Autodesk Inventor part; units mm, degrees
ref_plane "YZ Plane" through (0, 0, 0) normal (1, 0, 0) x (0, 1, 0)
ref_plane "XZ Plane" through (0, 0, 0) normal (0, 1, 0) x (-1, 0, 0)
ref_plane "XY Plane" through (0, 0, 0) normal (0, 0, 1) x (1, 0, 0)
sketch "Sketch1" plane through (0, 0, 0) normal (0, 0, 1) x (1, 0, 0)
  line L0 (0, 0) -> (25.4, 0)
  line L1 (25.4, 0) -> (25.4, 25.4)
  line L2 (25.4, 25.4) -> (0, 25.4)
  line L3 (0, 25.4) -> (0, 0)
  line L4 (1.5875, 1.5875) -> (23.8125, 1.5875)
  line L5 (23.8125, 1.5875) -> (23.8125, 23.8125)
  line L6 (23.8125, 23.8125) -> (1.5875, 23.8125)
  line L7 (1.5875, 23.8125) -> (1.5875, 1.5875)
  dimension "d0" = 25.4
  dimension "d1" = 25.4
  dimension "d2" = 1.5875
extrude "Extrusion1" add sketch "Sketch1" along normal blind 400.05
sketch "Sketch3" plane through (0, 25.4, 0) normal (0, 1, 0) x (1, 0, 0)
  line L0 (25.4, 0) -> (0, 0)
  line L1 (0, 0) -> (0, -400.05)
  line L2 (25.4, -400.05) -> (0, -400.05)
  line L3 (25.4, 0) -> (25.4, -400.05)
  point P0 (0, 0)
  point P1 (12.7, -200.025)
  dimension "d15" = 200.025
  dimension "d16" = 400.05
  dimension "d17" = 12.7
hole "Hole2" at (12.7, 25.4, 200.025) direction (0, -1, 0) diameter 6.35 end through all
sketch "Sketch7" plane through (0, 25.4, 0) normal (0, 1, 0) x (1, 0, 0)
  line L0 (0, 0) -> (0, -400.05)
  line L1 (25.4, 0) -> (25.4, -400.05)
  line L2 (25.4, 0) -> (0, 0)
  line L3 (0, 0) -> (25.4, 0)
  line L4 (0, -200.025) -> (0, 0)
  line L5 (25.4, 0) -> (25.4, -200.025)
  line L6 (0, 0) -> (25.4, 0)
  arc A0 (25.4, -200.025) -> (0, -200.025) centre (12.7, -200.025) ccw
  line L7 (25.4, -400.05) -> (0, -400.05)
  circle A1 centre (12.7, -200.025) radius 3.175
  line L8 (25.4, 0) -> (0, 0)
  line L9 (0, 0) -> (0, -400.05)
  line L10 (25.4, -400.05) -> (0, -400.05)
  line L11 (25.4, 0) -> (25.4, -400.05)
extrude "Extrusion3" cut sketch "Sketch7" against normal blind 25.4 contours L2 L1 A0 L0
sketch "Sketch8" plane through (0, 25.4, 400.05) normal (0, 1, 0) x (1, 0, 0)
  line L0 (25.4, 0) -> (0, 0)
  line L1 (0, 200.025) -> (0, 0)
  point P0 (0, 400.05)
  point P1 (12.7, 12.7)
  point P2 (12.7, 31.75)
  point P3 (12.7, 50.8)
  dimension "d43" = 12.7
  dimension "d44" = 12.7
  dimension "d55" = 19.05
  dimension "d56" = 19.05
hole "Hole4" at (12.7, 25.4, 387.35) at (12.7, 25.4, 368.3) at (12.7, 25.4, 349.25) direction (0, -1, 0) diameter 4.8514 end through all
properties part number "CLB_036_FourPartScissorBarTop" material "Aluminum 6061"
Read the model definition and answer for the solid it produces. Units are mm, in the model's axes. A direction names the side the tool comes from. Round coordinates to 2 decimals unless told otherwise and drop trailing zeros. Order: outer loops, then holes, each group sorted by start corner. A loop starts at its lowest first (then second) coordinate and runs counter-clockwise, first axis right, second up.
1) For faces 1 (the face through (13, 1.588, 292)), 2 (the face through (13, 25.4, 292)), determine the directions among +Z, -Z, +X, -X, +Y, -Y from which every point of the face is accessible in a straight line to the end or side of a thin tool.
2) The mould has two halves that part along Z. Classify faces 3 (the face through (1, 13, 400.05)), 4 (the face through (12.593, 0.783, 384.927)), 5 (the face through (1.588, 13, 296)), 6 (the face through (25.253, 15.7, 198.095)): released by +Z, released by -Z, zero draft, split by the parting line, or undercut.
3) A flat-ended cylindrical pin translates along its axis: pin 1 (3 mm diameter, centred on x = 17, y = 5, fed in from +Z). Find the tip coordinate at first contact, or state that the pin passes through.
4) The part is cut by section B-B on z = 344. Write down the section's boundary in (x, y).
5) The part is cut by section C-C on x = 12.7. Give the number of separate pieces and of enclosed holes in the cut face, plus the area to 3 significant figures.
6) Straight lines are drawn through the part: L1, parallel to Z at x = 12.7, y = 0.85 (3 decimals); L2, parallel to X at y = 15.75, z = 349.5. For each, find the intervals that lie inside material, in ascending order.
Resolved:
1. face 1: +Z, -Z
1. face 2: +Z, -Z, +X, -X, +Y
2. face 3: released by +Z
2. face 4: undercut
2. face 5: zero draft
2. face 6: released by -Z
3. pin 1: passes through
4. outline: (0, 0) - (25.4, 0) - (25.4, 25.4) - (0, 25.4) - close; hole (1.59, 1.59) - (23.81, 1.59) - (23.81, 23.81) - (1.59, 23.81) - close
5. separate pieces: 10
5. enclosed holes: 0
5. area: 609 mm2
6. L1: z = 187.325 to 196.85, 203.2 to 346.824, 351.676 to 365.874, 370.726 to 384.924, 389.776 to 400.05
6. L2: x = 0 to 1.59, 23.81 to 25.4
